For this review, take the finished solid that the model builds, in its own axes (mm). A direction names the side the tool comes from. Coordinates: 2 decimals unless noted, no trailing zeros. Loops run counter-clockwise (first coordinate to the right, second up) from the corner with the lowest first, then second, coordinate; pieces in that order, holes last. Notation, with made-up numbers: (56, 23) -> (72, 23) arc R13 ccw to (72, 30) -> close; hole circle Ø5 at (37.5, -12.75). An arc over 180 degrees is marked (long way). One line per item, written item: value.
from build123d import *

# Parameters (mm, degrees)
F0_R          = 43
F1_DEPTH      = 25
F5_R          = 4
F6_DEPTH      = 20
F6_DEPTH_BACK = 79
F4_R          = 4
F7_DEPTH      = 20
F7_DEPTH_BACK = 80
F3_R          = 4
F8_DEPTH      = 93.1
F8_DEPTH_BACK = 25
F2_R          = 4
F9_DEPTH      = 82.3
F9_DEPTH_BACK = 25


with BuildPart() as f1:
    # F0 (on Top) → F1 (new body)
    with BuildSketch(Plane.XY):
        Circle(F0_R)
        Polygon((-32.9113515503, 2.4172172296), (-21.5626091646, 24.9810705538), (2.4172172296, 32.9113515503), (24.9810705538, 21.5626091646), (32.9113515503, -2.4172172296), (21.5626091646, -24.9810705538), (-2.4172172296, -32.9113515503), (-24.9810705538, -21.5626091646), align=None, mode=Mode.SUBTRACT)
    extrude(amount=F1_DEPTH)

    # F5 (on face) → F6 (cut, two sides)
    with BuildSketch(Plane(origin=(-13.6991438917, -27.2369803574, 0), x_dir=(-0.8933665181, 0.4493286818, 0), z_dir=(0.4493286818, 0.8933665181, 0))) as f6_sk:
        with Locations((0, 12.5)):
            Circle(F5_R)
    extrude(amount=-F6_DEPTH, mode=Mode.SUBTRACT)
    extrude(f6_sk.sketch, amount=F6_DEPTH_BACK, mode=Mode.SUBTRACT)

    # F4 (on face) → F7 (cut, two sides)
    with BuildSketch(Plane(origin=(-28.946211052, -9.5726959675, 0), x_dir=(-0.3139821652, 0.9494288809, 0), z_dir=(0.9494288809, 0.3139821652, 0))) as f7_sk:
        with Locations((0, 12.5)):
            Circle(F4_R)
    extrude(amount=-F7_DEPTH, mode=Mode.SUBTRACT)
    extrude(f7_sk.sketch, amount=F7_DEPTH_BACK, mode=Mode.SUBTRACT)

    # F3 (on face) → F8 (cut, two sides)
    with BuildSketch(Plane(origin=(-27.2369803574, 13.6991438917, 0), x_dir=(0.4493286818, 0.8933665181, 0), z_dir=(0.8933665181, -0.4493286818, 0))) as f8_sk:
        with Locations((0, 12.5)):
            Circle(F3_R)
    extrude(amount=F8_DEPTH, mode=Mode.SUBTRACT)
    extrude(f8_sk.sketch, amount=-F8_DEPTH_BACK, mode=Mode.SUBTRACT)

    # F2 (on face) → F9 (cut, two sides)
    with BuildSketch(Plane(origin=(-9.5726959675, 28.946211052, 0), x_dir=(0.9494288809, 0.3139821652, 0), z_dir=(0.3139821652, -0.9494288809, 0))) as f9_sk:
        with Locations((0, 12.5)):
            Circle(F2_R)
    extrude(amount=F9_DEPTH, mode=Mode.SUBTRACT)
    extrude(f9_sk.sketch, amount=-F9_DEPTH_BACK, mode=Mode.SUBTRACT)


solid = f1.part
1. Take a section at C-C, the plane x = 4. Give the boundary of the cut face in (y, z).
Return value:
outline: (-42.81, 0) -> (-30.79, 0) -> (-30.79, 25) -> (-42.81, 25) -> close; (32.12, 0) -> (42.81, 0) -> (42.81, 25) -> (32.12, 25) -> close
2. Insertion check: pin 1 Ø3 at (y, z) = (6, 13) entering from +X; pin 2 Ø3 at (y, z) = (-27, 16.5) entering from -X; pin 3 Ø8 at (y, z) = (32, 16) entering from -X. Each pin has a flat end and moves straight along its axis. Give the tip position at first contact, or say it passes through.
Return value:
pin 1: stops at x = 42.76
pin 2: stops at x = -34.62
pin 3: stops at x = -32.63
3. Take a section at B-B, the plane z = 6.25. Give the boundary of the cut face in (x, y).
Return value:
outline: circle Ø86 at (0, 0); hole (-32.91, 2.42) -> (-24.98, -21.56) -> (-2.42, -32.91) -> (21.56, -24.98) -> (32.91, -2.42) -> (24.98, 21.56) -> (2.42, 32.91) -> (-21.56, 24.98) -> close
4. Take a section at A-A, the plane y = 0. Give the boundary of the cut face in (x, z), and give its area (3 significant figures).
Return value:
outline: (-43, 0) -> (-32.11, 0) -> (-32.11, 25) -> (-43, 25) -> close; (32.11, 0) -> (43, 0) -> (43, 25) -> (32.11, 25) -> close
area: 544 mm2
5. For faces 4 (the flat face through (28.58, -11.03, 9.55)), 5 (the cylindrical face through (-12.005, 34.642, 16.466)), list the 3-axis set-ups (+Z, -Z, +X, -X, +Y, -Y) from which the entire face can be reached by the end or side of a thin tool; tool diameter is ignored.
Return value:
face 4: +Z, -Z
face 5: none
6. The part is to be moulded in two halves that separate along Y. For faces 1 (the flat face through (-29.3, -9, 25)), 2 (the cylindrical face through (-42.96, 1.89, 12.32)), 3 (the cylindrical face through (34.46, -13.06, 13.7)), say which applies: pulls with the +Y half, pulls with the -Y half, needs draft (parallel to the pull), parting line crosses it, or undercut.
Return value:
face 1: needs draft
face 2: parting line crosses it
face 3: undercut
7. Take a section at D-D, the plane y = -13. Give the number of separate pieces and of enclosed holes in the cut face, and give its area (3 significant figures).
Return value:
separate pieces: 3
enclosed holes: 0
area: 532 mm2
8. To check wall thickness, follow probe 1 along Y at (x, z) = (29.5, 12); probe 2 along X at (y, z) = (37.5, 13.5); probe 3 along Y at (x, z) = (17, 19.25). State the ranges of each line that lie inside material, in increasing order. Write a range as from..to.
Return value:
probe 1: y = -31.28..-19.28, -10.4..-9.2, 13.94..31.28
probe 2: x = -21.04..-16.48, -8.32..14.53
probe 3: y = -39.5..-26.49, 25.58..39.5
